Build history of the part. All positions in model axes, mm. A direction names the side the tool comes from. Coordinates: 2 decimals unless noted, no trailing zeros. Order: outer loops, then holes, each group sorted by start corner. A loop starts at its lowest first (then second) coordinate and runs counter-clockwise, first axis right, second up. Notation, with made-up numbers: (35.5, 8) - (60.5, 8) arc R19 cw to (60.5, 34) - close; hole circle Ø2 at (-19, 22). An arc over 180 degrees is marked (long way). One line per item, written item: value.
Autodesk Inventor part; units mm, degrees
ref_plane "Work Plane1" through (0, 0, 9.8) normal (0, 0, 1) x (1, 0, 0)
ref_plane "Work Plane2" through (-147.35, 31.7362, 13.0715) normal (0, 0.1305262, 0.9914449) x (1, 0, 0)
ref_plane "Work Plane3" through (-145.35, -54.1, -1.5) normal (0, 0, 1) x (1, 0, 0)
ref_plane "Work Plane1" through (0, 0, 9.8) normal (0, 0, 1) x (1, 0, 0)
sketch "Sketch1" plane through (0, 0, 9.8) normal (0, 0, 1) x (1, 0, 0)
  line L0 (145.35, 54.1) -> (-145.35, 54.1)
  line L1 (145.35, -54.1) -> (145.35, 54.1)
  line L2 (-145.35, -54.1) -> (145.35, -54.1)
  line L3 (-145.35, 54.1) -> (-145.35, -54.1)
  line L4 (143.1, 53.975) -> (-143.1, 53.975)
  line L5 (-143.1, 53.975) -> (-143.1, -51.85)
  line L6 (-143.1, -51.85) -> (143.1, -51.85)
  line L7 (143.1, -51.85) -> (143.1, 53.975)
  point P0 (0, 0)
  dimension "d0" = 0.125
  dimension "d1" = 2.25
  dimension "d2" = 2.25
  dimension "d3" = 2.25
ref_plane "Work Plane2" through (-147.35, 31.7362, 13.0715) normal (0, 0.1305262, 0.9914449) x (1, 0, 0)
extrude "Extrusion1" add sketch "Sketch1" along normal up to surface contours L7 L6 L5 L4 surface through (-147.35, 31.7362, 13.0715) normal (0, 0.1305262, 0.9914449)
sketch "Sketch3" plane through (0, 0, 9.8) normal (0, 0, -1) x (-1, 0, 0)
  line L0 (143.1, 48.1) -> (-143.1, 48.1)
  line L1 (-143.1, -51.85) -> (-143.1, 53.975)
  line L2 (-143.1, -48.1) -> (143.1, -48.1)
  line L3 (143.1, 53.975) -> (143.1, -51.85)
  line L4 (-143.1, 53.975) -> (143.1, 53.975)
  line L5 (143.1, -51.85) -> (-143.1, -51.85)
  point P0 (0, 0)
  dimension "d8" = 5.875
  dimension "d9" = 3.75
ref_plane "Work Plane3" through (-145.35, -54.1, -1.5) normal (0, 0, 1) x (1, 0, 0)
extrude "Extrusion2" add sketch "Sketch3" along normal up to surface (11.3 mm away) contours L0 L1 L4 L3 | L3 L5 L1 L2
sketch "Sketch4" plane through (-143.1, -48.1, 9.8) normal (-1, 0, 0) x (0, 0, 1)
  line L0 (14.2758, -3.75) -> (0.3437, 102.075)
  line L1 (13.3027, 3.6417) -> (1.7, -3.75)
  line L2 (-11.3, -3.75) -> (14.2758, -3.75)
  line L3 (0.7, -6) -> (0.7, -8)
  point P0 (-9.8, 48.1)
  dimension "d12" = 65
  dimension "d23" = 1
extrude "Extrusion3" cut sketch "Sketch4" against normal through all
sketch "Sketch5" plane through (-143.1, -51.85, -1.5) normal (0, -1, 0) x (1, 0, 0)
  line L0 (0, 13) -> (0, 24.6027)
  line L1 (0, 13) -> (5.4104, 24.6027)
  line L2 (0, 24.6027) -> (286.2, 24.6027)
  point P0 (143.1, 1.5)
  dimension "d15" = 65
sketch "Sketch6" plane through (-143.1, -48.1, 9.8) normal (-1, 0, 0) x (0, 0, 1)
  line L0 (1.7, -3.75) -> (3.3295, 79.3957)
  point P0 (-9.8, 48.1)
  point P1 (0.3437, 102.075)
  dimension "d16" = 22.875
sweep "Sweep1" cut profiles "Sketch5" path "Sketch6"
mirror "Mirror1" about plane through (0, 0, 0) normal (1, 0, 0) of "Sweep1"
ref_plane "Work Plane4" through (-143.1, 53.7139, 8.1608) normal (0, 0.1305262, 0.9914449) x (1, 0, 0)
sketch "Sketch8" plane through (-143.1, 53.975, 10.1437) normal (0, 0.1305262, 0.9914449) x (1, 0, 0)
  line L0 (286.2, 0) -> (286.2, -22.875)
  line L1 (286.2, -15) -> (0, -15)
  line L2 (0, -22.875) -> (0, 0)
  line L3 (0, 0) -> (286.2, 0)
  point P0 (143.1, -52.1892)
  dimension "d20" = 15
extrude "Extrusion4" add sketch "Sketch8" against normal up to surface (2 mm away)
sketch "Sketch9" plane through (-143.1, -51.85, -1.5) normal (0, -1, 0) x (1, 0, 0)
  line L0 (286.2, 0) -> (286.2, 11.6437)
  line L1 (286.2, 3) -> (0, 3)
  line L2 (0, 10.3999) -> (0, 0)
  line L3 (286.2, 0) -> (0, 0)
  point P0 (143.1, 1.5)
  dimension "d24" = 3
properties part number "bottom"
1. Band-saw the part on B-B, the plane x = 15.5. Give the cut face in (y, z) (3 decimals).
Values found:
outline: (-51.85, -1.5) - (-48.1, -1.5) - (-48.1, 9.8) - (41.263, 9.8) - (48.1, 8.9) - (48.1, -1.5) - (53.975, -1.5) - (53.975, 10.144) - (-44.458, 23.103) - (-51.85, 11.5) - close
2. 3-axis set-ups, long thin cutter, end or side, ignore diameter. For faces 5 (the face through (-2, -51.85, 5)), 6 (the face through (-2, -3, 9.8)): which of +Z, -Z, +X, -X, +Y, -Y reach the whole face in a straight line?
Values found:
face 5: +Z, -Z, +X, -X, -Y
face 6: -Z, +X, -X
3. Band-saw the part on D-D, the plane z = 20. Give the cut face in (x, y), and give its area (3 significant figures).
Values found:
outline: (-139.42, -20.89) - (-139.19, -46.43) - (139.19, -46.43) - (139.42, -20.89) - close
area: 7,120 mm2
4. Probe line 1 along Y through (x, z) = (-64, 3) (3 decimals); line 2 along Z through (x, y) = (-115.5, -47); line 3 along X through (y, z) = (-41, 15). List the from-to ranges inside material, lowest first.
Values found:
line 1: y = -51.85 to -48.1, 48.1 to 53.975
line 2: z = 9.8 to 19.11
line 3: x = -141.57 to 141.57
5. Flat gauge pins, fed straight in: P1, Ø1, axis at x = 106, y = 27.5, coming from the +Z side; P2, Ø5, axis at x = -58, y = 10, coming from the +Z side; P3, Ø6, axis at x = 82, y = 15.5, coming from the +Z side. Where does each tip first touch, or does it go through?
Values found:
P1: stops at z = 13.7
P2: stops at z = 16.26
P3: stops at z = 15.6
6. Band-saw the part on A-A, the plane z = 2. Give the cut face in (x, y) (3 decimals).
Values found:
outline: (-143.1, -51.85) - (143.1, -51.85) - (143.1, -48.1) - (-143.1, -48.1) - close; (-143.1, 48.1) - (143.1, 48.1) - (143.1, 53.975) - (-143.1, 53.975) - close
7. Band-saw the part on C-C, the plane y = -32. Give the cut face in (x, z).
Values found:
outline: (-143.1, 9.8) - (143.1, 9.8) - (143.1, 11.89) - (138.64, 21.46) - (-138.64, 21.46) - (-143.1, 11.89) - close
8. Two-plate mould, pull along Y, no slides. Class faces 1 (the face through (-2, 48.1, 4)), 2 (the face through (-2.003, 4.069, 16.714)), 3 (the face through (143.1, 1, 10)), 4 (the face through (-2.003, 44.729, 9.344)): pulls with the +Y half, pulls with the -Y half, needs draft (parallel to the pull), parting line crosses it, or undercut.
Values found:
face 1: undercut
face 2: pulls with the +Y half
face 3: needs draft
face 4: undercut
